Autodesk Inventor part; units mm, degrees
ref_plane "YZ Plane" through (0, 0, 0) normal (1, 0, 0) x (0, 1, 0)
ref_plane "XZ Plane" through (0, 0, 0) normal (0, 1, 0) x (-1, 0, 0)
ref_plane "XY Plane" through (0, 0, 0) normal (0, 0, 1) x (1, 0, 0)
sketch "Esquisse1" plane through (0, 0, 0) normal (0, 1, 0) x (-1, 0, 0)
  line L0 (-20, 65) -> (20, 65)
  line L1 (20, 65) -> (20, -65)
  line L2 (20, -65) -> (-20, -65)
  line L3 (-20, -65) -> (-20, 65)
  line L4 (-20, 65) -> (20, -65) construction
  line L5 (20, 65) -> (-20, -65) construction
  point P0 (0, 0)
  dimension "d0" = 40
  dimension "d1" = 130
extrude "Extrusion1" add sketch "Esquisse1" along normal mid plane 90
sketch "Esquisse2" plane through (20, 45, -65) normal (0, 0, -1) x (-1, 0, 0)
  line L0 (0, 0) -> (40, 0)
  line L1 (16, 0) -> (16, -7)
  line L2 (16, -7) -> (12, -7)
  line L3 (12, -7) -> (12, -15)
  line L4 (20, 0.6313) -> (20, -19.069)
  line L5 (12, -15) -> (20, -15)
  line L6 (24, 0) -> (24, -7)
  line L7 (24, -7) -> (28, -7)
  line L8 (28, -7) -> (28, -15)
  line L9 (28, -15) -> (20, -15)
  point P0 (20, -45)
  point P1 (20, 0)
  dimension "d4" = 7
  dimension "d5" = 4
  dimension "d6" = 4
  dimension "d7" = 8
extrude "Extrusion2" cut sketch "Esquisse2" against normal through all
sketch "Esquisse3" plane through (-20, -45, 65) normal (0, 0, 1) x (1, 0, 0)
  line L0 (40, 0) -> (40, 90)
  line L1 (0, 25) -> (40, 25)
  line L2 (40, 25) -> (40, 0)
  line L3 (40, 0) -> (0, 0)
  line L4 (0, 0) -> (0, 25)
  line L5 (0, 25) -> (40, 0) construction
  line L6 (40, 25) -> (0, 0) construction
  point P0 (20, 45)
  point P1 (20, 12.5)
  dimension "d10" = 25
extrude "Extrusion3" add sketch "Esquisse3" along normal blind 30
fillet "Congé1" radius 2 6 edges at (20, -20, 80) (20, -32.5, 95) (0, -20, 95) (-20, -20, 80) (-20, -32.5, 95) (0, -45, 95)
sketch "Esquisse4" plane through (-18, -20, 65) normal (0, 1, 0) x (1, 0, 0)
  line L0 (0, -28) -> (0, 0)
  line L1 (36, -28) -> (0, -28)
  line L2 (36, 0) -> (36, -28)
  line L3 (0, 0) -> (36, 0)
  line L4 (46, 65) -> (-10, 65)
  point P0 (18, 65)
  point P1 (18.2732, -10)
  dimension "d21" = 75
hole "Perçage1" at (0.2732, -20, 75) direction (0, -1, 0) diameter 16 end through all
mirror "Mise en miroir2" about plane through (0, 0, 0) normal (0, 0, 1) of "Extrusion3", "Congé1", "Perçage1"
properties part number "Support"
Could you check a few things on this model? Use its own coordinates, in mm. A direction names the side the tool comes from. Give positions to 0.01 mm unless a question says otherwise; leave off trailing zeros. Write each loop counter-clockwise with the first axis right and the second up, starting at its lowest first coordinate (ties: lowest second). Pieces come first, ordered by that corner, then holes. Notation, with made-up numbers: (44.5, 62) -> (80.5, 62) arc R22 ccw to (80.5, 77) -> close; hole circle Ø9 at (20.25, -20). An arc over 180 degrees is marked (long way). Write each question's results on one line, items separated by ' | '. Start each with the question number.
Q1. I'm going to push flat-ended pins straight in: pin 1 Ø4 at (x, y) = (-12.5, 19.5) entering from +Z; pin 2 Ø14 at (x, z) = (-7, -80.5) entering from +Y; pin 3 Ø5 at (x, z) = (2, 21) entering from +Y; pin 4 Ø8 at (x, y) = (7, 3) entering from -Z. Where does each tip first touch, or does it pass through?
Q2. We'd pull the mould along X, two halves only. Please class faces 5 (the face through (12, 45, 1)), 6 (the face through (20, 1, 1)), 7 (the face through (6, 38, -1)): +X half, -X half, draft (parallel to the pull), parting line (faces both ways), or undercut.
Q3. Suppose I cut it at C-C, the plane z = -4. List the corners of the cut face in (x, y) for me.
Q4. I need wall thicknesses on probe 1 along Z at (x, y) = (-5, -31.5); probe 2 along Y at (x, z) = (7.5, 30); probe 3 along X at (y, z) = (-39.5, -75). Which ranges of each line are inside material? Lowest first, please.
Q5. Suppose I cut it at A-A, the plane z = -75. List the corners of the cut face in (x, y) for me, and give its area (3 significant figures).
Q6. Which directions (+Z, -Z, +X, -X, +Y, -Y) give clear straight access to the entire face, cutting with the end or side of a thin tool? Please do faces 1 (the face through (-4, 42, -1)), 2 (the face through (0, 30, -1)), 3 (the face through (0, -20, -85)), 4 (the face through (-4, -20, 82)).
Q7. Suppose I cut it at D-D, the plane y = -33. List the corners of the cut face in (x, z) for me, and give its area (3 significant figures).
Q8. Suppose I cut it at B-B, the plane x = -15.5. List the corners of the cut face in (y, z) for me.
Outcome:
1) pin 1: z = 65 | pin 2: y = -20 | pin 3: y = 45 | pin 4: z = -65
2) face 5: draft | face 6: +X half | face 7: undercut
3) outline: (-20, -45) -> (20, -45) -> (20, 45) -> (4, 45) -> (4, 38) -> (8, 38) -> (8, 30) -> (-8, 30) -> (-8, 38) -> (-4, 38) -> (-4, 45) -> (-20, 45) -> close
4) probe 1: -95 to -81.02, -68.98 to 68.98, 81.02 to 95 | probe 2: -45 to 30, 38 to 45 | probe 3: -20 to -7.73, 8.27 to 20
5) outline: (-20, -45) -> (-7.73, -45) -> (-7.73, -20) -> (-18, -20) arc R2 ccw to (-20, -22) -> close; (8.27, -45) -> (20, -45) -> (20, -22) arc R2 ccw to (18, -20) -> (8.27, -20) -> close | area: 598 mm2
6) face 1: +Z, -Z, +Y | face 2: +Z, -Z | face 3: -Z, +X, -X, +Y | face 4: +Z, +X, -X, +Y
7) outline: (-20, -93) arc R2 ccw to (-18, -95) -> (18, -95) arc R2 ccw to (20, -93) -> (20, 93) arc R2 ccw to (18, 95) -> (-18, 95) arc R2 ccw to (-20, 93) -> close; hole circle Ø16 at (0.27, -75); hole circle Ø16 at (0.27, 75) | area: 7,190 mm2
8) outline: (-45, -93) arc R2 ccw to (-43, -95) -> (-22, -95) arc R2 ccw to (-20, -93) -> (-20, -65) -> (45, -65) -> (45, 65) -> (-20, 65) -> (-20, 93) arc R2 ccw to (-22, 95) -> (-43, 95) arc R2 ccw to (-45, 93) -> close
